from build123d import *

# Parameters (mm, degrees)
SKETCH_1_R      = 1.25
SKETCH_1_R_2    = 1.500000003
SKETCH_1_R_3    = 1.500000002
EXTRUDE_1_DEPTH = 3


with BuildPart() as part:
    # 草圖1 → 填料-伸長1 (new body)
    with BuildSketch(Plane.XY):
        with BuildLine():
            Line((88.500524103, 145.700017948), (35.000524103, 145.700292307))
            ThreePointArc((35.000524103, 145.700292307), (32.879119595, 144.821703189), (32.000508719, 142.700307692))
            Line((32.000508719, 142.700307692), (32.000300001, 99.000307693))
            ThreePointArc((32.000300001, 99.000307693), (32.878839121, 96.878853187), (35.000284616, 96.000292308))
            Line((35.000284616, 96.000292308), (89.000284615, 96.000015385))
            ThreePointArc((89.000284615, 96.000015385), (91.121639122, 96.878654505), (92.0003, 99))
            Line((92.0003, 99), (92.000408718, 142.7))
            ThreePointArc((92.000408718, 142.7), (91.121779951, 144.82129415), (89.000524103, 145.700015384))
            Line((89.000524103, 145.700015384), (88.500524103, 145.700017948))
        make_face()
        with Locations((52.50039487, 117.000202566)):
            Circle(SKETCH_1_R, mode=Mode.SUBTRACT)
        with Locations((52.500297434, 99.000202566)):
            Circle(SKETCH_1_R, mode=Mode.SUBTRACT)
        with Locations((36.500451283, 128.500284615)):
            Circle(SKETCH_1_R_2, mode=Mode.SUBTRACT)
        with Locations((62.000492306, 136.500153847)):
            Circle(SKETCH_1_R_3, mode=Mode.SUBTRACT)
        Polygon((84.824140487, 116.000036801), (84.824089205, 106.000036801), (81.824089205, 106.000052186), (81.824140487, 116.000052185), align=None, mode=Mode.SUBTRACT)
        Polygon((64.000315385, 102.00014359), (64.000376923, 114.00014359), (41.000376924, 114.000261539), (41.000315385, 102.000261539), align=None, mode=Mode.SUBTRACT)
        Polygon((38.000402565, 119.000276923), (35.000402565, 119.000292308), (35.000433334, 125.000292308), (38.000433334, 125.000276923), align=None, mode=Mode.SUBTRACT)
        Polygon((38.000469231, 132.000276923), (35.000469231, 132.000292308), (35.000500001, 138.000292308), (38.000500001, 138.000276923), align=None, mode=Mode.SUBTRACT)
        Polygon((39.500500001, 138.000269231), (39.500484616, 135.000269231), (49.500484616, 135.000217948), (49.500500001, 138.000217948), align=None, mode=Mode.SUBTRACT)
        Polygon((74.500484616, 135.000089743), (84.500484615, 135.000038461), (84.5005, 138.000038461), (74.5005, 138.000089743), align=None, mode=Mode.SUBTRACT)
    extrude(amount=EXTRUDE_1_DEPTH)


solid = part.part
The listing builds one solid part. Answer for the finished solid, in the listing's coordinates (mm). Give positions to 0.01 mm unless a question says otherwise; leave off trailing zeros. Order: outer loops, then holes, each group sorted by start corner. A loop starts at its lowest first (then second) coordinate and runs counter-clockwise, first axis right, second up. Notation, with made-up numbers: (64, 78.25) - (75, 78.25) arc R15 ccw to (75, 87.25) - close; hole circle Ø7 at (65.5, 63). An arc over 180 degrees is marked (long way). Use one line per item in the form item = value.
1) Find section B-B on y = 122.5. Determine the outline of the cut face in (x, z), and give its area (3 significant figures).
Verdict:
outline = (32, 0) - (35, 0) - (35, 3) - (32, 3) - close; (38, 0) - (92, 0) - (92, 3) - (38, 3) - close
area = 171 mm^2
2) Find section D-D on y = 109.5. Determine the outline of the cut face in (x, z), and give its area (3 significant figures).
Verdict:
outline = (32, 0) - (41, 0) - (41, 3) - (32, 3) - close; (64, 0) - (81.82, 0) - (81.82, 3) - (64, 3) - close; (84.82, 0) - (92, 0) - (92, 3) - (84.82, 3) - close
area = 102 mm^2
3) Consider probe 1 along Y at (x, z) = (82, 2.3); probe 2 along Y at (x, z) = (49, 1.25); probe 3 along X at (y, z) = (109, 1.5). Determine where each line is inside the solid, lowest interval first. Write a range as [from, to].
Verdict:
probe_1 = [96, 106], [116, 135], [138, 145.7]
probe_2 = [96, 102], [114, 135], [138, 145.7]
probe_3 = [32, 41], [64, 81.82], [84.82, 92]
4) Find section A-A on x = 79. Determine the outline of the cut face in (y, z), and give its area (3 significant figures).
Verdict:
outline = (96, 0) - (135, 0) - (135, 3) - (96, 3) - close; (138, 0) - (145.7, 0) - (145.7, 3) - (138, 3) - close
area = 140 mm^2
5) Find section C-C on x = 52.5. Determine the outline of the cut face in (y, z).
Verdict:
outline = (96, 0) - (97.75, 0) - (97.75, 3) - (96, 3) - close; (100.25, 0) - (102, 0) - (102, 3) - (100.25, 3) - close; (114, 0) - (115.75, 0) - (115.75, 3) - (114, 3) - close; (118.25, 0) - (145.7, 0) - (145.7, 3) - (118.25, 3) - close
